Source: three-view drawing plus pictorial views. Frame: mm from the lowest corner of the part. A direction names the side the tool comes from. Round coordinates to 2 decimals unless told otherwise and drop trailing zeros. Order: outer loops, then holes, each group sorted by start corner. A loop starts at its lowest first (then second) coordinate and runs counter-clockwise, first axis right, second up. Notation, with made-up numbers: (80, 17.5) -> (134, 17.5) arc R21 ccw to (134, 21.5) -> close; hole circle Ø2 at (-35.5, 85.5). An arc over 180 degrees is marked (long way). Use a Markdown table: item, result.
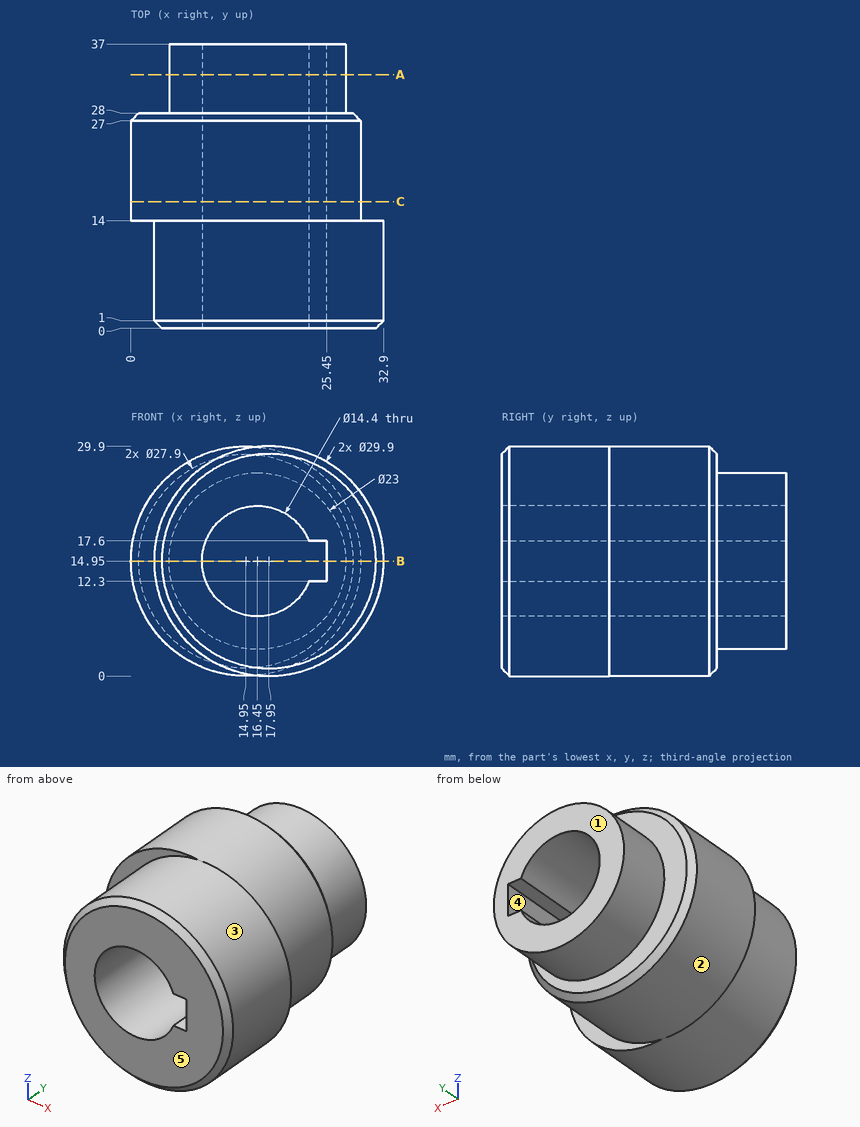
1) Pin query (flat end, axial travel): pin 1 Ø1.5 at (y, z) = (6.5, 6) entering from +X; pin 2 Ø1.6 at (y, z) = (27.5, 14.5) entering from -X; pin 3 Ø8 at (x, y) = (24.5, 19) entering from +Z; pin 4 Ø8 at (x, y) = (23.5, 29.5) entering from -Z. Return the tip coordinate at first contact, or that it passes through.
Results found:
| item | result |
|---|---|
| pin 1 | stops at x = 30.45 |
| pin 2 | stops at x = 0 |
| pin 3 | stops at z = 28.83 |
| pin 4 | stops at z = 1.02 |
2) Cut plane C-C on y = 16.5. Return loops of the section in (x, z).
Results found:
| item | result |
|---|---|
| outline | circle Ø29.9 at (14.95, 14.95); hole (23.14, 12.3) -> (25.45, 12.3) -> (25.45, 17.6) -> (23.14, 17.6) arc R7.2 ccw (long way) to start |
3) Line query: L1, parallel to X at y = 19, z = 14.95; L2, parallel to X at y = 11, z = 14.95; L3, parallel to Z at x = 15, y = 33. Output: solid intervals per line, ascending. Write a range as [from, to].
Results found:
| item | result |
|---|---|
| L1 | x = [0, 9.25], [25.45, 29.9] |
| L2 | x = [3, 9.25], [25.45, 32.9] |
| L3 | z = [3.54, 7.9], [22, 26.36] |
4) Set-up query: the marked faces 1, 2, 3, 4 and 5. Return all of +Z, -Z, +X, -X, +Y, -Y with unobstructed straight access to the full face (end or side cutting, diameter ignored); none if empty.
Results found:
| item | result |
|---|---|
| face 1 | +Z, -Z, +X, -X, +Y |
| face 2 | +Y |
| face 3 | -Y |
| face 4 | +Y, -Y |
| face 5 | +Z, -Z, +X, -X, -Y |
5) Cut plane B-B on z = 14.95. Return loops of the section in (x, y), and give its area (3 significant figures).
Results found:
| item | result |
|---|---|
| outline | (0, 14) -> (3, 14) -> (3, 1) -> (4, 0) -> (9.25, 0) -> (9.25, 37) -> (4.95, 37) -> (4.95, 28) -> (1, 28) -> (0, 27) -> close; (25.45, 0) -> (31.9, 0) -> (32.9, 1) -> (32.9, 14) -> (29.9, 14) -> (29.9, 27) -> (28.9, 28) -> (27.95, 28) -> (27.95, 37) -> (25.45, 37) -> close |
| area | 443 mm² |
6) Cut plane A-A on y = 33. Return loops of the section in (x, z).
Results found:
| item | result |
|---|---|
| outline | circle Ø23 at (16.45, 14.95); hole (23.14, 12.3) -> (25.45, 12.3) -> (25.45, 17.6) -> (23.14, 17.6) arc R7.2 ccw (long way) to start |
